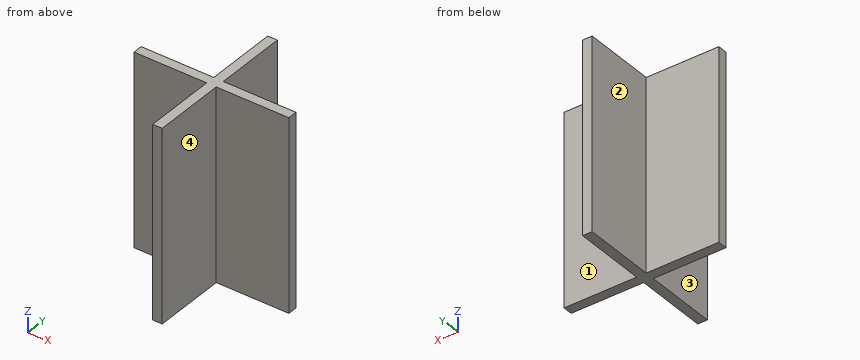
from build123d import *

# Parameters (mm, degrees)
F0_W     = 380
F0_H     = 50
F0_W_2   = 50
F0_H_2   = 380
F1_DEPTH = 1000


with BuildPart() as f1:
    # F0 (on Top) → F1 (new body)
    with BuildSketch(Plane.XY):
        with Locations((-216.727231, -26.01678)):
            Rectangle(F0_W, F0_H)
        with Locations((213.272769, -26.01678)):
            Rectangle(F0_W, F0_H)
        with Locations((-1.727231, 188.98322)):
            Rectangle(F0_W_2, F0_H_2)
        Polygon((0, -51.01678), (-26.727231, -51.01678), (-26.727231, -431.01678), (23.272769, -431.01678), (23.272769, -51.01678), align=None)
        Polygon((23.272769, -1.01678), (-26.727231, -1.01678), (-26.727231, -51.01678), (0, -51.01678), (23.272769, -51.01678), align=None)
    extrude(amount=F1_DEPTH)


solid = f1.part
Work out the finished part from the listing and answer in its coordinate system (mm). Face numbers are marked on the shaded views. A direction names the side the tool comes from. Round coordinates to 2 decimals unless told otherwise and drop trailing zeros. Loops run counter-clockwise (first coordinate to the right, second up) from the corner with the lowest first, then second, coordinate; pieces in that order, holes last. Notation, with made-up numbers: (7, 49.5) -> (27, 49.5) arc R18 ccw to (27, 56.5) -> close; hole circle Ø4 at (-22, 1). An arc over 180 degrees is marked (long way). Use one line per item in the form item = value.
(1) Straight lines are drawn through the part: line 1 (Y direction, x = -268, z = 76); line 2 (X direction, y = -135, z = 665). For each, find the intervals that lie inside material, in ascending order.
Answer list:
line_1 = -51.02 to -1.02
line_2 = -26.73 to 23.27
(2) Find section A-A on z = 694. Give the vertices of the cut face in (x, y).
Answer list:
outline = (-406.73, -51.02) -> (-26.73, -51.02) -> (-26.73, -431.02) -> (23.27, -431.02) -> (23.27, -51.02) -> (403.27, -51.02) -> (403.27, -1.02) -> (23.27, -1.02) -> (23.27, 378.98) -> (-26.73, 378.98) -> (-26.73, -1.02) -> (-406.73, -1.02) -> close
(3) A tool of negligible diameter and unlimited length cuts with its end or side. For the marked faces 1, 2, 3 and 4, from which of +Z, -Z, +X, -X, +Y, -Y can it reach the whole face along a straight path? Write none if from no direction.
Answer list:
face_1 = +Z, -Z, +X, +Y
face_2 = +Z, -Z, -X, +Y
face_3 = +Z, -Z, -X, -Y
face_4 = +Z, -Z, +X, -Y
(4) Find section C-C on x = 63. Give the vertices of the cut face in (y, z).
Answer list:
outline = (-51.02, 0) -> (-1.02, 0) -> (-1.02, 1000) -> (-51.02, 1000) -> close
(5) Flat-ended cylindrical pins translate along their axes: P1, Ø6, axis at y = -92, z = 174, coming from the +X side; P2, Ø2, axis at y = -119, z = 420, coming from the -X side; P3, Ø2, axis at x = 215, z = 462.5, coming from the -Y side. Find the tip coordinate at first contact, or state that the pin passes through.
Answer list:
P1 = 23.27
P2 = -26.73
P3 = -51.02
(6) Find section B-B on y = 111. Give the vertices of the cut face in (x, z), then the cut area to 3 significant figures.
Answer list:
outline = (-26.73, 0) -> (23.27, 0) -> (23.27, 1000) -> (-26.73, 1000) -> close
area = 50,000 mm2
